The model under review builds one solid part; all positions refer to its coordinate system, in mm. Round coordinates to 2 decimals unless told otherwise and drop trailing zeros. Write each loop counter-clockwise with the first axis right and the second up, starting at its lowest first coordinate (ties: lowest second). Pieces come first, ordered by that corner, then holes. Notation, with made-up numbers: (74.5, 68.25) -> (112.5, 68.25) arc R14 ccw to (112.5, 88.25) -> close; hole circle Ø10 at (60.25, -34). An arc over 180 degrees is marked (long way). Return JSON: item names as keys, results as strings. Group by question number.
1. Take a section at C-C, the plane x = 20. Write out the cut boundary in (y, z).
2. Take a section at B-B, the plane y = 3.75. Write out the cut boundary in (x, z).
3. Take a section at A-A, the plane z = 0. Write out the cut boundary in (x, y).
4. Mouldability with a two-part tool opening along Z and no side actions: class faces 1 (the cylindrical face through (-18.414, 2.712, -0.208)), 2 (the cylindrical face through (-24.43, 2.79, 6.9)), 3 (the flat face through (25, 3, 0)) as pulls with the +Z half, pulls with the -Z half, needs draft (parallel to the pull), parting line crosses it, or undercut.
5. For line 1 along X through (y, z) = (4.3, 0); line 2 along Z through (x, y) = (-0.5, 2.3); line 3 along X through (y, z) = (1.8, -6.5), list the stretches that pass through material, from the lowest coordinate up. Write a range as from..to.
6. Clearance check with a flat-ended pin moving along its axis: P1, Ø5, axis at x = -20, z = 0, coming from the -Y side. State where the tip first meets the part, or that it passes through.
7. Take a section at D-D, the plane x = -21. Write out the cut boundary in (y, z), then the cut area to 3 significant figures.
from build123d import *

# Parameters (mm, degrees)
SKETCH_1_W      = 50
SKETCH_1_H      = 15
SKETCH_1_R      = 1.6
EXTRUDE_1_DEPTH = 5.5
FILLET_1_R      = 2


with BuildPart() as part:
    # 草图1 → 凸台-拉伸1 (new body)
    with BuildSketch(Plane(origin=(0, 0, 0), x_dir=(1, 0, 0), z_dir=(0, 1, 0))):
        Rectangle(SKETCH_1_W, SKETCH_1_H)
        with Locations(Location((-20, 0, 0), (0, 0, 270))):
            Circle(SKETCH_1_R, mode=Mode.SUBTRACT)
        with Locations(Location((0, 0, 0), (0, 0, 270))):
            Circle(SKETCH_1_R, mode=Mode.SUBTRACT)
        with Locations(Location((20, 0, 0), (0, 0, 270))):
            Circle(SKETCH_1_R, mode=Mode.SUBTRACT)
    extrude(amount=EXTRUDE_1_DEPTH)

    # 圆角1
    fillet_1_edges = [part.edges().sort_by_distance(p)[0] for p in [
        (25, 2.75, 7.5),
        (-25, 2.75, 7.5),
        (-25, 2.75, -7.5),
        (25, 2.75, -7.5),
    ]]
    fillet(fillet_1_edges, radius=FILLET_1_R)


solid = part.part
Output:
{
 "1": {"outline": "(0, -7.5) -> (5.5, -7.5) -> (5.5, -1.6) -> (0, -1.6) -> close; (0, 1.6) -> (5.5, 1.6) -> (5.5, 7.5) -> (0, 7.5) -> close"},
 "2": {"outline": "(-25, -5.5) arc R2 ccw to (-23, -7.5) -> (23, -7.5) arc R2 ccw to (25, -5.5) -> (25, 5.5) arc R2 ccw to (23, 7.5) -> (-23, 7.5) arc R2 ccw to (-25, 5.5) -> close; hole circle Ø3.2 at (-20, 0); hole circle Ø3.2 at (0, 0); hole circle Ø3.2 at (20, 0)"},
 "3": {"outline": "(-25, 0) -> (-21.6, 0) -> (-21.6, 5.5) -> (-25, 5.5) -> close; (-18.4, 0) -> (-1.6, 0) -> (-1.6, 5.5) -> (-18.4, 5.5) -> close; (1.6, 0) -> (18.4, 0) -> (18.4, 5.5) -> (1.6, 5.5) -> close; (21.6, 0) -> (25, 0) -> (25, 5.5) -> (21.6, 5.5) -> close"},
 "4": {"face 1": "undercut", "face 2": "pulls with the +Z half", "face 3": "needs draft"},
 "5": {"line 1": "x = -25..-21.6, -18.4..-1.6, 1.6..18.4, 21.6..25", "line 2": "z = -7.5..-1.52, 1.52..7.5", "line 3": "x = -24.73..24.73"},
 "6": {"P1": "stops at y = 0"},
 "7": {"outline": "(0, -7.5) -> (5.5, -7.5) -> (5.5, -1.25) -> (0, -1.25) -> close; (0, 1.25) -> (5.5, 1.25) -> (5.5, 7.5) -> (0, 7.5) -> close", "area": "68.8 mm^2"}
}
